Can you work these out from the drawing? Everything is in mm from the part's minimum corner. Give positions to 0.01 mm unless a question says otherwise; leave off trailing zeros. Loops run counter-clockwise (first coordinate to the right, second up) from the corner with the lowest first, then second, coordinate; pieces in that order, holes last. Notation, with made-up numbers: M 17.25,6.25 L 44.25,6.25 A27 ccw 44.25,42.25 Z; hole C 35,-29.75 d10. An arc over 180 degrees is marked long. Use CSV: the item, a comma, the result in double quotes.
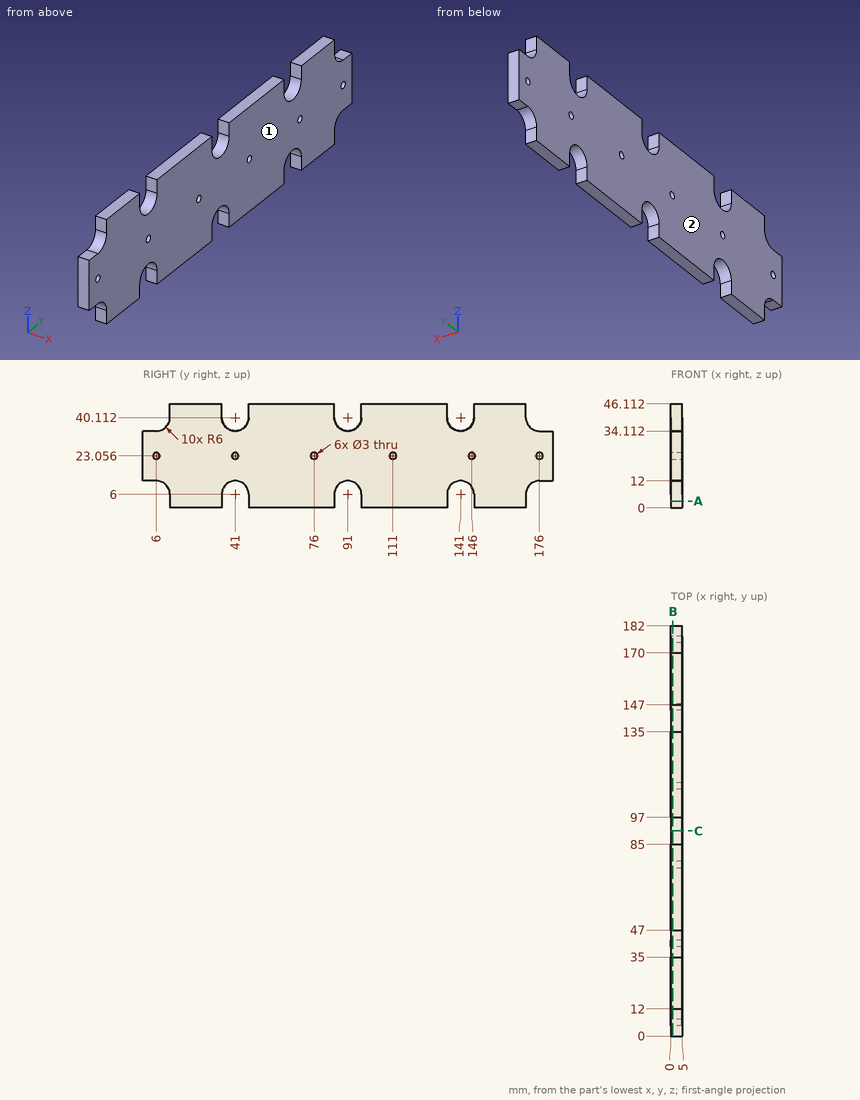
Q1. I want a section at B-B, the plane x = 0.9. State how many separate pieces and enclosed holes the cut face has, then the cut area to 3 significant figures.
Model answer:
separate pieces,"1"
enclosed holes,"6"
area,"7,030 mm2"
Q2. I want a section at C-C, the plane y = 91. Please give me the cut outline in (x, z).
Model answer:
outline,"M 0,12 L 5,12 L 5,34.11 L 0,34.11 Z"
Q3. I want a section at A-A, the plane z = 3. Please give me the cut outline in (x, y), then the cut area to 3 significant figures.
Model answer:
outline,"M 0,12 L 5,12 L 5,35 L 0,35 Z; M 0,47 L 5,47 L 5,85 L 0,85 Z; M 0,97 L 5,97 L 5,135 L 0,135 Z; M 0,147 L 5,147 L 5,170 L 0,170 Z"
area,"610 mm2"
Q4. Please list where these lines run through material, in increasing order: L1, parallel to Y at x = 2.3, z = 2; L2, parallel to Y at x = 3.75, z = 36; L3, parallel to Z at x = 2.75, y = 76. Write a range as from..to.
Model answer:
L1,"12..35, 47..85, 97..135, 147..170"
L2,"10.37..36.63, 45.37..86.63, 95.37..136.63, 145.37..171.63"
L3,"0..21.56, 24.56..46.11"
Q5. If we mould it in two halves opening along X, with no side actions, what happens to the marked faces 1 and 2? For each: released by +X, released by -X, zero draft, split by the parting line, or undercut.
Model answer:
face 1,"released by +X"
face 2,"released by -X"
Q6. I'm going to push flat-ended pins straight in: P1, Ø2.5, axis at x = 2, z = 42.5, coming from the -Y side; P2, Ø2.5, axis at x = 1.5, z = 43, coming from the +Y side; P3, Ø2.5, axis at x = 1.5, y = 3.5, coming from the +Z side; P4, Ø2.5, axis at y = 6, z = 23.056, coming from the +X side. Where does each tip first touch, or does it pass through?
Model answer:
P1,"y = 12"
P2,"y = 170"
P3,"z = 34.11"
P4,"through"
